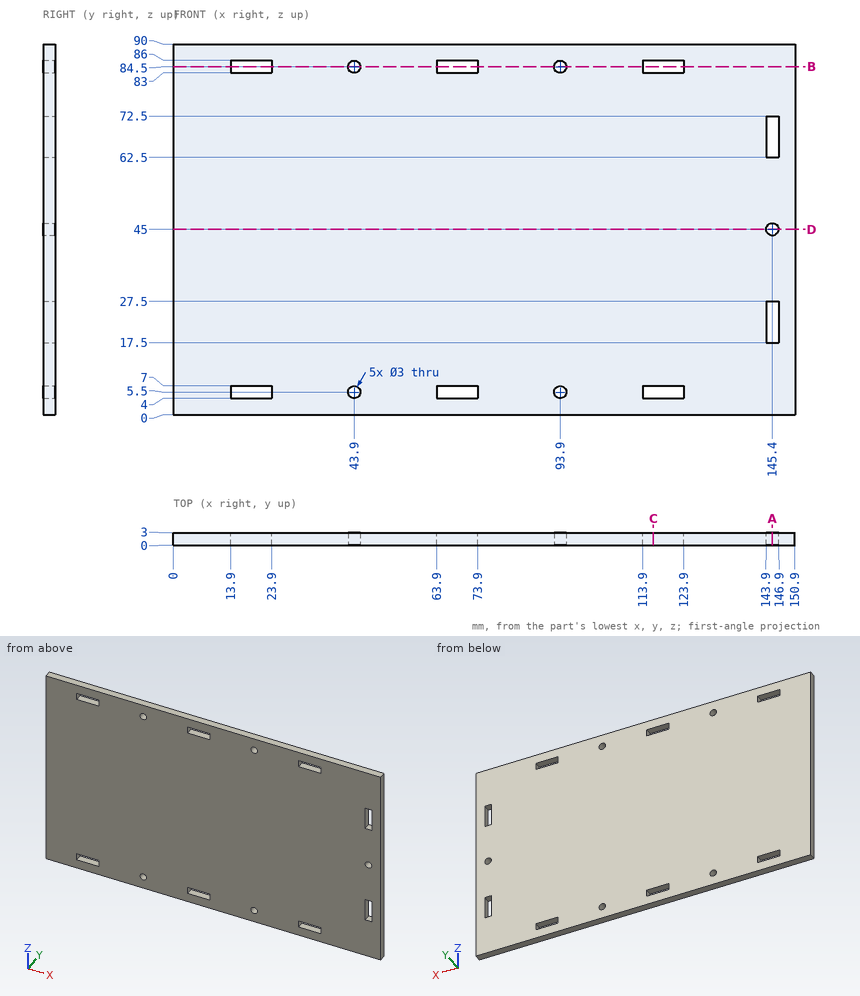
Part print with two shaded views. Sizes in mm from the minimum x, y, z corner. Give positions to 0.01 mm unless a question says otherwise; leave off trailing zeros. Write each loop counter-clockwise with the first axis right and the second up, starting at its lowest first coordinate (ties: lowest second). Pieces come first, ordered by that corner, then holes.
1) Pin check, flat tip, straight feed: pin 1 (1.5 mm diameter, centred on x = 68.5, y = 1.5, fed in from -Z). Stop position of the tip, or through.
Resolved:
pin 1: stops at z = 0
2) Cut at D-D on z = 45. Write the cut outline in (x, y).
Resolved:
outline: (0, 0) - (143.9, 0) - (143.9, 3) - (0, 3) - close; (146.9, 0) - (150.9, 0) - (150.9, 3) - (146.9, 3) - close
3) Probe L1, parallel to X at y = 0.7, z = 84.5; L2, parallel to Z at x = 93.9, y = 1.35; L3, parallel to X at y = 2.3, z = 19. List the from-to ranges inside material, lowest first.
Resolved:
L1: x = 0 to 13.9, 23.9 to 42.4, 45.4 to 63.9, 73.9 to 92.4, 95.4 to 113.9, 123.9 to 150.9
L2: z = 0 to 4, 7 to 83, 86 to 90
L3: x = 0 to 143.9, 146.9 to 150.9
4) Cut at A-A on x = 145.4. Write the cut outline in (y, z), then the cut area to 3 significant figures.
Resolved:
outline: (0, 0) - (3, 0) - (3, 17.5) - (0, 17.5) - close; (0, 27.5) - (3, 27.5) - (3, 43.5) - (0, 43.5) - close; (0, 46.5) - (3, 46.5) - (3, 62.5) - (0, 62.5) - close; (0, 72.5) - (3, 72.5) - (3, 90) - (0, 90) - close
area: 201 mm2
5) Cut at C-C on x = 116.5. Write the cut outline in (y, z).
Resolved:
outline: (0, 0) - (3, 0) - (3, 4) - (0, 4) - close; (0, 7) - (3, 7) - (3, 83) - (0, 83) - close; (0, 86) - (3, 86) - (3, 90) - (0, 90) - close
6) Cut at B-B on z = 84.5. Write the cut outline in (x, y), then the cut area to 3 significant figures.
Resolved:
outline: (0, 0) - (13.9, 0) - (13.9, 3) - (0, 3) - close; (23.9, 0) - (42.4, 0) - (42.4, 3) - (23.9, 3) - close; (45.4, 0) - (63.9, 0) - (63.9, 3) - (45.4, 3) - close; (73.9, 0) - (92.4, 0) - (92.4, 3) - (73.9, 3) - close; (95.4, 0) - (113.9, 0) - (113.9, 3) - (95.4, 3) - close; (123.9, 0) - (150.9, 0) - (150.9, 3) - (123.9, 3) - close
area: 345 mm2
